The listing builds one solid part. Answer for the finished solid, in the listing's coordinates (mm). Round coordinates to 2 decimals unless told otherwise and drop trailing zeros. Loops run counter-clockwise (first coordinate to the right, second up) from the corner with the lowest first, then second, coordinate; pieces in that order, holes last. Notation, with made-up numbers: (-37.5, -1.5) -> (13.5, -1.5) arc R22 ccw to (13.5, 37.5) -> close; hole circle Ø8 at (-7.5, -35). An arc over 180 degrees is marked (long way). Write each question's results on one line, items separated by ' | '. Start each with the question number.
(1) A flat-ended cylindrical pin translates along its axis: pin 1 (2.5 mm diameter, centred on x = -27, y = 0, fed in from +Z). Find the tip coordinate at first contact, or state that the pin passes through.
(2) The part is cut by section A-A (x = 0). Determine the outline of the cut face in (y, z).
(3) Straight lines are drawn through the part: probe 1 along Y at (x, z) = (12.5, 1.4); probe 2 along Y at (x, z) = (26.5, 0.65); probe 3 along X at (y, z) = (8.5, 0.95). For each, find the intervals that lie inside material, in ascending order.
(4) The part is cut by section B-B (y = -27). Determine the outline of the cut face in (x, z), plus the area to 3 significant figures.
(5) The part is cut by section D-D (z = 1.05). Count the separate pieces of the cut face and the enclosed holes in it, plus the area to 3 significant figures.
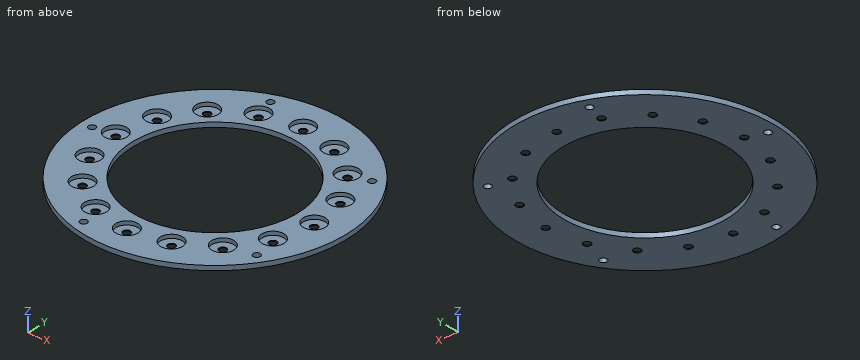
```python
from build123d import *

# Parameters (mm, degrees)
SKETCH1_R           = 35
BOSS_EXTRUDE1_DEPTH = 1.55
SKETCH2_R           = 22
CUT_EXTRUDE1_DEPTH  = 50.521737651
SKETCH3_R           = 2.95
CUT_EXTRUDE6_DEPTH  = 1
SKETCH5_R           = 1
CUT_EXTRUDE7_DEPTH  = 50.521737651
MOVE_FACE1_BY       = 0.3
CIRPATTERN2_COUNT   = 16
SKETCH6_R           = 0.95
CUT_EXTRUDE8_DEPTH  = 50.513255801
CIRPATTERN3_COUNT   = 5


with BuildPart() as part:
    # Sketch1 → Boss-Extrude1 (new body)
    with BuildSketch(Plane.XY):
        Circle(SKETCH1_R)
    extrude(amount=BOSS_EXTRUDE1_DEPTH)

    # Sketch2 → Cut-Extrude1 (cut, through all)
    with BuildSketch(Plane.XY.offset(1.55)):
        Circle(SKETCH2_R)
    extrude(amount=-CUT_EXTRUDE1_DEPTH, mode=Mode.SUBTRACT)

    # Sketch3 → Cut-Extrude6 (cut)
    with BuildSketch(Plane.XY.offset(1.55)):
        with Locations((0, 27)):
            Circle(SKETCH3_R)
    cut_extrude6 = extrude(amount=-CUT_EXTRUDE6_DEPTH, mode=Mode.SUBTRACT)

    # Sketch5 → Cut-Extrude7 (cut, through all)
    with BuildSketch(Plane.XY.offset(1.55)):
        with Locations((0, 27)):
            Circle(SKETCH5_R)
    cut_extrude7 = extrude(amount=-CUT_EXTRUDE7_DEPTH, mode=Mode.SUBTRACT)

    # Move Face1: a face moved inward by 0.3
    extrude(part.faces().sort_by_distance((0, -28, 0))[0], amount=MOVE_FACE1_BY, dir=(0, 0, 1), mode=Mode.SUBTRACT)

    # CirPattern2: Cut-Extrude6, Cut-Extrude7 ×16 about axis
    cirpattern2_axis = Axis((0, 0, 0), (0, 0, 1))
    add([cut_extrude6.rotate(cirpattern2_axis, i * 360 / CIRPATTERN2_COUNT) for i in range(1, CIRPATTERN2_COUNT)], mode=Mode.SUBTRACT)
    add([cut_extrude7.rotate(cirpattern2_axis, i * 360 / CIRPATTERN2_COUNT) for i in range(1, CIRPATTERN2_COUNT)], mode=Mode.SUBTRACT)

    # Sketch6 → Cut-Extrude8 (cut, through all)
    with BuildSketch(Plane(origin=(0, 0, 0.3), x_dir=(-1, 0, 0), z_dir=(0, 0, -1))):
        with Locations((11.467774385, 29.874573648)):
            Circle(SKETCH6_R)
    cut_extrude8 = extrude(amount=-CUT_EXTRUDE8_DEPTH, mode=Mode.SUBTRACT)

    # CirPattern3: Cut-Extrude8 ×5 about axis
    cirpattern3_axis = Axis((0, 0, 0), (0, 0, 1))
    for i in range(1, CIRPATTERN3_COUNT):
        add(cut_extrude8.rotate(cirpattern3_axis, i * 360 / CIRPATTERN3_COUNT), mode=Mode.SUBTRACT)


solid = part.part
```
Checked values:
1) pin 1: stops at z = 0.55
2) outline: (-35, 0.3) -> (-28, 0.3) -> (-28, 0.55) -> (-29.95, 0.55) -> (-29.95, 1.55) -> (-35, 1.55) -> close; (-26, 0.3) -> (-22, 0.3) -> (-22, 1.55) -> (-24.05, 1.55) -> (-24.05, 0.55) -> (-26, 0.55) -> close; (22, 0.3) -> (26, 0.3) -> (26, 0.55) -> (24.05, 0.55) -> (24.05, 1.55) -> (22, 1.55) -> close; (28, 0.3) -> (35, 0.3) -> (35, 1.55) -> (29.95, 1.55) -> (29.95, 0.55) -> (28, 0.55) -> close
3) probe 1: y = -32.69 to -26.95, -22.94 to -18.1, 18.1 to 22.94, 26.95 to 32.69 | probe 2: y = -22.86 to -18.32, -16.54 to -12.84, -7.83 to -2.91, 2.91 to 7.83, 12.84 to 22.86 | probe 3: x = -33.95 to -27.26, -22.63 to -20.29, 20.29 to 22.63, 27.26 to 33.95
4) outline: (-22.27, 0.3) -> (-1, 0.3) -> (-1, 0.55) -> (-2.95, 0.55) -> (-2.95, 1.55) -> (-8.22, 1.55) -> (-8.22, 0.55) -> (-12.45, 0.55) -> (-12.45, 1.55) -> (-22.27, 1.55) -> close; (1, 0.3) -> (22.27, 0.3) -> (22.27, 1.55) -> (12.45, 1.55) -> (12.45, 0.55) -> (8.22, 0.55) -> (8.22, 1.55) -> (2.95, 1.55) -> (2.95, 0.55) -> (1, 0.55) -> close | area: 40.8 mm2
5) separate pieces: 1 | enclosed holes: 22 | area: 1,880 mm2
